Check sheet for the modelled part. Datum: model origin and axes. Units: mm. Give positions to 0.01 mm unless a question says otherwise; leave off trailing zeros. Order: outer loops, then holes, each group sorted by start corner. A loop starts at its lowest first (then second) coordinate and runs counter-clockwise, first axis right, second up.
```python
from build123d import *

# Parameters (mm, degrees)
SKETCH2_R             = 4
SKETCH2_R_2           = 2.00000381
BOSS_EXTRUDE1_DEPTH   = 5
BOSS_EXTRUDE1_2_DEPTH = 5
BOSS_EXTRUDE1_3_DEPTH = 5
BOSS_EXTRUDE1_4_DEPTH = 5
BOSS_EXTRUDE2_DEPTH   = 2
FILLET1_R             = 15
CUT_EXTRUDE1_REACH    = 4
SKETCH4_R             = 1.75
CHAMFER1_SIZE         = 1


with BuildPart() as part:
    # Sketch2 → Boss-Extrude1 (new body)
    with BuildSketch(Plane(origin=(0, 0, 183.407141652), x_dir=(-1, 0, 0), z_dir=(0, 0, -1))):
        with Locations((-136.154543014, 230.793193515)):
            Circle(SKETCH2_R)
        with Locations((-136.154543014, 230.793193515)):
            Circle(SKETCH2_R_2, mode=Mode.SUBTRACT)
    extrude(amount=BOSS_EXTRUDE1_DEPTH)



with BuildPart() as body_2:
    # Sketch2 → Boss-Extrude1 2 (new body)
    with BuildSketch(Plane(origin=(0, 0, 183.407141652), x_dir=(-1, 0, 0), z_dir=(0, 0, -1))):
        with Locations((-44.154357594, 230.793193515)):
            Circle(SKETCH2_R)
        with Locations((-44.154357594, 230.793193515)):
            Circle(SKETCH2_R_2, mode=Mode.SUBTRACT)
    extrude(amount=BOSS_EXTRUDE1_2_DEPTH)


with BuildPart() as body_3:
    # Sketch2 → Boss-Extrude1 3 (new body)
    with BuildSketch(Plane(origin=(0, 0, 183.407141652), x_dir=(-1, 0, 0), z_dir=(0, 0, -1))):
        with Locations((-44.154357594, 138.793008095)):
            Circle(SKETCH2_R)
        with Locations((-44.154357594, 138.793008095)):
            Circle(SKETCH2_R_2, mode=Mode.SUBTRACT)
    extrude(amount=BOSS_EXTRUDE1_3_DEPTH)


with BuildPart() as body_4:
    # Sketch2 → Boss-Extrude1 4 (new body)
    with BuildSketch(Plane(origin=(0, 0, 183.407141652), x_dir=(-1, 0, 0), z_dir=(0, 0, -1))):
        with Locations((-136.154543014, 138.793008095)):
            Circle(SKETCH2_R)
        with Locations((-136.154543014, 138.793008095)):
            Circle(SKETCH2_R_2, mode=Mode.SUBTRACT)
    extrude(amount=BOSS_EXTRUDE1_4_DEPTH)


with BuildPart() as part_1:
    add(part.part)

    add(body_2.part)  # Boss-Extrude2 merges body 2

    add(body_3.part)  # Boss-Extrude2 merges body 3

    add(body_4.part)  # Boss-Extrude2 merges body 4
    # Sketch3 → Boss-Extrude2 (add)
    with BuildSketch(Plane(origin=(0, 0, 178.407141652), x_dir=(-1, 0, 0), z_dir=(0, 0, -1))):
        with BuildLine():
            Line((-139.007032023, 227.989034737), (-115.141850609, 184.935107777))
            Line((-115.141850609, 184.935107777), (-139.523599689, 140.949268079))
            ThreePointArc((-139.523599689, 140.949268079), (-138.922212365, 135.905101177), (-133.857043766, 135.518638354))
            Line((-133.857043766, 135.518638354), (-90.042023818, 159.8057005))
            Line((-90.042023818, 159.8057005), (-46.919036743, 135.902238439))
            ThreePointArc((-46.919036743, 135.902238439), (-41.612813753, 135.704229226), (-40.785300919, 140.949268079))
            Line((-40.785300919, 140.949268079), (-65.167049999, 184.935107777))
            Line((-65.167049999, 184.935107777), (-41.301868585, 227.989034737))
            ThreePointArc((-41.301868585, 227.989034737), (-41.306554913, 233.602111436), (-46.919036743, 233.683963171))
            Line((-46.919036743, 233.683963171), (-90.042023818, 209.78050111))
            Line((-90.042023818, 209.78050111), (-133.857043766, 234.067563256))
            ThreePointArc((-133.857043766, 234.067563256), (-139.206449083, 233.378898322), (-139.007032023, 227.989034737))
        make_face()
    extrude(amount=-BOSS_EXTRUDE2_DEPTH)

    # Fillet1
    fillet1_edges = [part_1.edges().sort_by_distance(p)[0] for p in [
        (90.042023818, 209.78050111, 179.407141652),
        (65.167049999, 184.935107777, 179.407141652),
        (90.042023818, 159.8057005, 179.407141652),
        (115.141850609, 184.935107777, 179.407141652),
    ]]
    fillet(fillet1_edges, radius=FILLET1_R)

    # Sketch4 → Cut-Extrude1 (cut, up to next)
    with BuildSketch(Plane.XY.offset(180.407141652), mode=Mode.PRIVATE) as cut_extrude1_sk1:
        with Locations((70.167049999, 204.78050111)):
            Circle(SKETCH4_R)
    cut_extrude1_tool1 = extrude(cut_extrude1_sk1.sketch, amount=-CUT_EXTRUDE1_REACH, mode=Mode.PRIVATE) & part_1.part
    add(cut_extrude1_tool1.solids().sort_by_distance((70.16705, 204.780501, 180.407142))[0], mode=Mode.SUBTRACT)
    # Sketch4 → Cut-Extrude1 (cut, up to next)
    with BuildSketch(Plane.XY.offset(180.407141652), mode=Mode.PRIVATE) as cut_extrude1_sk2:
        with Locations((110.141850609, 204.78050111)):
            Circle(SKETCH4_R)
    cut_extrude1_tool2 = extrude(cut_extrude1_sk2.sketch, amount=-CUT_EXTRUDE1_REACH, mode=Mode.PRIVATE) & part_1.part
    add(cut_extrude1_tool2.solids().sort_by_distance((110.141851, 204.780501, 180.407142))[0], mode=Mode.SUBTRACT)
    # Sketch4 → Cut-Extrude1 (cut, up to next)
    with BuildSketch(Plane.XY.offset(180.407141652), mode=Mode.PRIVATE) as cut_extrude1_sk3:
        with Locations((110.141850609, 164.8057005)):
            Circle(SKETCH4_R)
    cut_extrude1_tool3 = extrude(cut_extrude1_sk3.sketch, amount=-CUT_EXTRUDE1_REACH, mode=Mode.PRIVATE) & part_1.part
    add(cut_extrude1_tool3.solids().sort_by_distance((110.141851, 164.805701, 180.407142))[0], mode=Mode.SUBTRACT)
    # Sketch4 → Cut-Extrude1 (cut, up to next)
    with BuildSketch(Plane.XY.offset(180.407141652), mode=Mode.PRIVATE) as cut_extrude1_sk4:
        with Locations((70.167049999, 164.8057005)):
            Circle(SKETCH4_R)
    cut_extrude1_tool4 = extrude(cut_extrude1_sk4.sketch, amount=-CUT_EXTRUDE1_REACH, mode=Mode.PRIVATE) & part_1.part
    add(cut_extrude1_tool4.solids().sort_by_distance((70.16705, 164.805701, 180.407142))[0], mode=Mode.SUBTRACT)

    # Chamfer1
    chamfer1_edges = [part_1.edges().sort_by_distance(p)[0] for p in [
        (68.417049999, 164.8057005, 180.407141652),
        (108.391850609, 164.8057005, 180.407141652),
        (108.391850609, 204.78050111, 180.407141652),
        (68.417049999, 204.78050111, 180.407141652),
    ]]
    chamfer(chamfer1_edges, length=CHAMFER1_SIZE)


solid = part_1.part
```
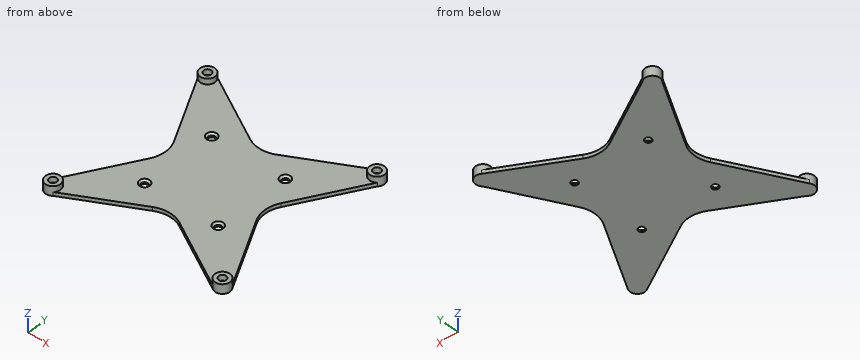
(1) Gauge pin test, flat ends, axial feed: pin 1 Ø3 at (y, z) = (177, 179.5) entering from -X; pin 2 Ø10 at (x, y) = (59, 145) entering from +Z; pin 3 Ø2 at (x, z) = (125, 179) entering from -Y. Record the tip position at first contact, or that the pin passes through.
Response values:
pin 1: stops at x = 59.94
pin 2: stops at z = 180.41
pin 3: stops at y = 139.87
(2) Cross-section at B-B on x = 55.5. Enter the section's corners in (y, z).
Response values:
outline: (140.66, 178.41) - (167.5, 178.41) - (167.5, 180.41) - (140.66, 180.41) - close; (202.37, 178.41) - (228.93, 178.41) - (228.93, 180.41) - (202.37, 180.41) - close
(3) Cross-section at C-C on y = 216.5. Enter the section's corners in (x, z).
Response values:
outline: (47.67, 178.41) - (77.92, 178.41) - (77.92, 180.41) - (47.67, 180.41) - close; (102.16, 178.41) - (132.64, 178.41) - (132.64, 180.41) - (102.16, 180.41) - close
(4) Cross-section at A-A on z = 181.65. Enter the section's corners in (x, y), then the cut area to 3 significant figures.
Response values:
outline: circle Ø8 at (44.15, 138.79); circle Ø8 at (44.15, 230.79); circle Ø8 at (136.15, 138.79); circle Ø8 at (136.15, 230.79); hole circle Ø4 at (44.15, 138.79); hole circle Ø4 at (44.15, 230.79); hole circle Ø4 at (136.15, 138.79); hole circle Ø4 at (136.15, 230.79)
area: 151 mm2
(5) Material ranges on L1, parallel to X at y = 155.5, z = 178.85; L2, parallel to Y at x = 50, z = 179.3; L3, parallel to Z at x = 87, y = 157.5, recorded low to high.
Response values:
L1: x = 48.85 to 82.27, 97.81 to 131.46
L2: y = 137.61 to 157.57, 212.3 to 231.98
L3: z = 178.41 to 180.41
(6) Cross-section at D-D on x = 99. Enter the section's corners in (y, z), then the cut area to 3 significant figures.
Response values:
outline: (154.84, 178.41) - (214.75, 178.41) - (214.75, 180.41) - (154.84, 180.41) - close
area: 120 mm2
